from build123d import *

# Parameters (mm, degrees)
F1_DEPTH = 3.175
F2_R     = 3.175
F3_DEPTH = 25.4


with BuildPart() as f1:
    # F0 (on Top) → F1 (new body)
    with BuildSketch(Plane.XY):
        Polygon((29.745836, 88.9), (-29.745836, 88.9), (-63.5, 48.554318), (-63.5, -48.554318), (-29.745836, -88.9), (29.745836, -88.9), (63.5, -48.554318), (63.5, 48.554318), align=None)
    extrude(amount=F1_DEPTH)

    # F2 (on face) → F3 (cut)
    with BuildSketch(Plane.XY.offset(3.175)):
        with Locations((-43.392069, 57.744911)):
            Circle(F2_R)
        with Locations((-35.242826, 67.48554)):
            Circle(F2_R)
        with Locations((35.242824, 67.485542)):
            Circle(F2_R)
        with Locations((43.392067, 57.744913)):
            Circle(F2_R)
        with Locations((43.392069, -57.744911)):
            Circle(F2_R)
        with Locations((35.242826, -67.48554)):
            Circle(F2_R)
        with Locations((-35.242826, -67.48554)):
            Circle(F2_R)
        with Locations((-43.392069, -57.744911)):
            Circle(F2_R)
    extrude(amount=-F3_DEPTH, mode=Mode.SUBTRACT)


solid = f1.part
Can you work these out from the model? Positions are in its coordinate system, mm. Give positions to 0.01 mm unless a question says otherwise; leave off trailing zeros. Loops run counter-clockwise (first coordinate to the right, second up) from the corner with the lowest first, then second, coordinate; pieces in that order, holes last. Notation, with made-up numbers: (50.25, -9.5) - (65.25, -9.5) arc R18 ccw to (65.25, 12.5) - close; hole circle Ø11 at (38, -28.5). An arc over 180 degrees is marked (long way). Answer as a JSON object with one key per item and string values.
Q1. Will this pin go through, and if not, where does the flat tip stop? P1, Ø5, axis at x = 43.39, y = 57.74, coming from the +Z side.
Geometry says:
{"P1": "through"}
Q2. If we mould it in two halves opening along Y, with no side actions, what happens to faces 1 (the cylindrical face through (32.07, 67.63, 1.61)), 2 (the flat face through (-1, 1, 0)), 3 (the flat face through (-46.859, -68.445, 1.565))? For each: pulls with the +Y half, pulls with the -Y half, needs draft (parallel to the pull), parting line crosses it, or undercut.
Geometry says:
{"face 1": "undercut", "face 2": "needs draft", "face 3": "pulls with the -Y half"}
Q3. Imagine slicing it at A-A on z = 1.75. Give the number of separate pieces and of enclosed holes in the cut face, plus the area to 3 significant figures.
Geometry says:
{"separate pieces": "1", "enclosed holes": "8", "area": "19,600 mm²"}
Q4. If I drill on L1, parallel to Y at x = 42, z = 2.95; L2, parallel to Y at x = 34.5, z = 2.2; L3, parallel to X at y = -65, z = 1.6, over which ranges is the centre line in solid material (lowest first)?
Geometry says:
{"L1": "-74.25 to -60.6, -54.89 to 54.89, 60.6 to 74.25", "L2": "-83.22 to -70.57, -64.4 to 64.4, 70.57 to 83.22", "L3": "-49.74 to -37.22, -33.27 to 33.27, 37.22 to 49.74"}
Q5. Imagine slicing it at B-B on x = 42. Write out the boundary of the cut face in (y, z) (3 decimals), plus the area to 3 significant figures.
Geometry says:
{"outline": "(-74.253, 0) - (-60.598, 0) - (-60.598, 3.175) - (-74.253, 3.175) - close; (-54.891, 0) - (54.891, 0) - (54.891, 3.175) - (-54.891, 3.175) - close; (60.598, 0) - (74.253, 0) - (74.253, 3.175) - (60.598, 3.175) - close", "area": "435 mm²"}
